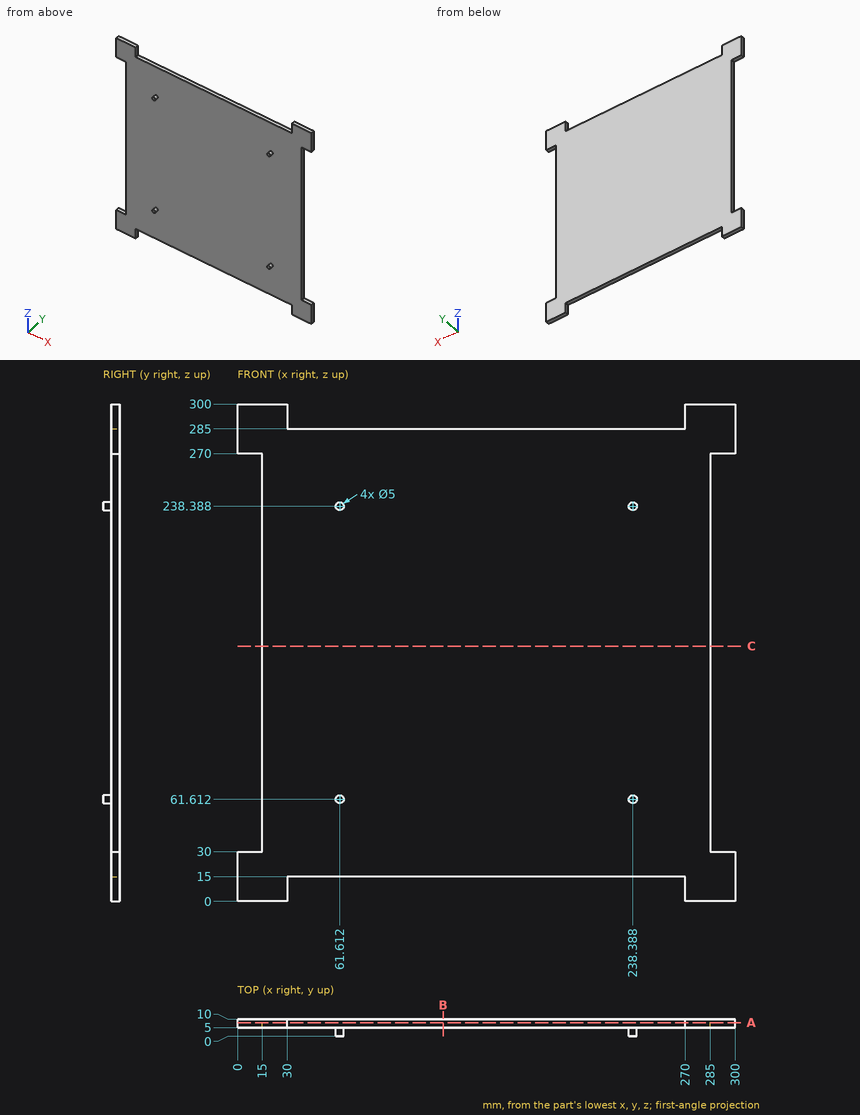
Geometry check sheet. Reference: drawing and pictorial views, mm from the part's lowest x, y, z. Coordinates: 2 decimals unless noted, no trailing zeros. Loops run counter-clockwise (first coordinate to the right, second up) from the corner with the lowest first, then second, coordinate; pieces in that order, holes last. Notation, with made-up numbers: (76.5, 20) -> (110.5, 20) arc R16 cw to (110.5, 47) -> close; hole circle Ø7 at (27.5, 5.25). An arc over 180 degrees is marked (long way). Write item = value, one per line. Start each with the question number.
1. Section check C-C on z = 154. Record the cut outline in (x, y).
2. Section check A-A on y = 8. Record the cut outline in (x, z).
3. Depth check by flat-ended pin: P1, Ø2.5, axis at x = 122, y = 7, coming from the -Z side; P2, Ø6, axis at y = 5.5, z = 142, coming from the -X side; P3, Ø3, axis at y = 8, z = 233, coming from the +X side. Enter the tip coordinate at first touch or a pass-through.
4. Material ranges on line 1 (Y direction, x = 149.5, z = 171.5); line 2 (X direction, y = 7.5, z = 155.5), recorded low to high.
5. Section check B-B on x = 124. Record the cut outline in (y, z).
Responses:
q1.outline = (15, 5) -> (285, 5) -> (285, 10) -> (15, 10) -> close
q2.outline = (0, 0) -> (30, 0) -> (30, 15) -> (270, 15) -> (270, 0) -> (300, 0) -> (300, 30) -> (285, 30) -> (285, 270) -> (300, 270) -> (300, 300) -> (270, 300) -> (270, 285) -> (30, 285) -> (30, 300) -> (0, 300) -> (0, 270) -> (15, 270) -> (15, 30) -> (0, 30) -> close
q3.P1 = 15
q3.P2 = 15
q3.P3 = 285
q4.line_1 = 5 to 10
q4.line_2 = 15 to 285
q5.outline = (5, 15) -> (10, 15) -> (10, 285) -> (5, 285) -> close
